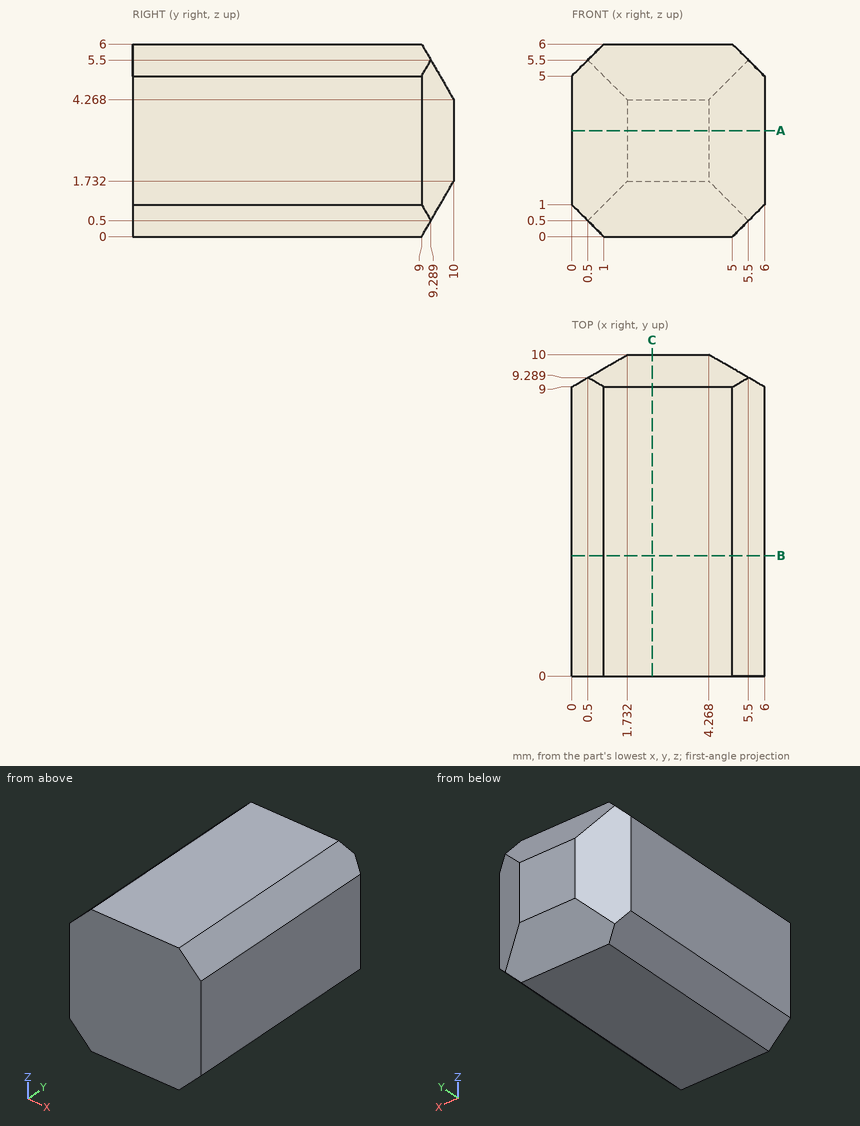
The figure shows three views and two pictorial views of one solid part (mm, origin at its lowest corner). Answer the questions. Round coordinates to 2 decimals unless told otherwise and drop trailing zeros. Write each loop counter-clockwise with the first axis right and the second up, starting at its lowest first coordinate (ties: lowest second). Pieces come first, ordered by that corner, then holes. Notation, with made-up numbers: (30, 4.5) - (61, 4.5) arc R9 ccw to (61, 9.5) - close; hole circle Ø4 at (48.5, -2). An arc over 180 degrees is marked (long way). Use one line per item in the form item = value. Start each with the question number.
Item 1: A cutting plane is placed at A-A (z = 3.3). Write down the section's boundary in (x, y).
Item 2: A cutting plane is placed at B-B (y = 3.75). Write down the section's boundary in (x, z), plus the area to 3 significant figures.
Item 3: A flat-ended cylindrical pin translates along its axis: pin 1 Ø1.5 at (x, z) = (3, 3.5) entering from -Y. Find the tip coordinate at first contact, or state that the pin passes through.
Item 4: A cutting plane is placed at C-C (x = 2.5). Write down the section's boundary in (y, z).
Item 5: Find the intervals of material crossed by line 1 (Y direction, x = 0.65, z = 4.2) (1 decimal); line 2 (Z direction, x = 3.55, y = 9.25) (1 decimal); line 3 (Y direction, x = 4.6, z = 0.3), in increasing order. Write a range as [from, to].
The answers:
q1.outline = (0, 0) - (6, 0) - (6, 9) - (4.27, 10) - (1.73, 10) - (0, 9) - close
q2.outline = (0, 1) - (1, 0) - (5, 0) - (6, 1) - (6, 5) - (5, 6) - (1, 6) - (0, 5) - close
q2.area = 34.0 mm^2
q3.pin_1 = 0
q4.outline = (0, 0) - (9, 0) - (10, 1.73) - (10, 4.27) - (9, 6) - (0, 6) - close
q5.line_1 = [0, 9.4]
q5.line_2 = [0.4, 5.6]
q5.line_3 = [0, 9.17]
